For this review, take the finished solid that the model builds, in its own axes (mm). A direction names the side the tool comes from. Coordinates: 2 decimals unless noted, no trailing zeros. Write each loop counter-clockwise with the first axis right and the second up, starting at its lowest first coordinate (ties: lowest second). Pieces come first, ordered by that corner, then holes. Notation, with made-up numbers: (-35, -22) - (-1, -22) arc R24 ccw to (-1, -8) - close; hole circle Ø11 at (-2.5, -2). An arc over 180 degrees is marked (long way). Write each question's results on one line, items separated by ' | '.
from build123d import *

# Parameters (mm, degrees)
F0_R           = 11.4851473357
F1_DEPTH       = 25.4
F2_R           = 14.0381408387
F3_DEPTH       = 38.354
F4_R           = 11.1184182472
F5_DEPTH       = 40.64
F6_R           = 11.1443418508
F7_DEPTH       = 25.4
F8_R           = 10.6779324927
F9_DEPTH       = 25.4
F10_W          = 48.1841601431
F10_H          = 38.3043847978
F11_DEPTH      = 13.97
F11_DEPTH_BACK = 13.97
F12_W          = 27.94
F12_H          = 23.4013380416
F13_DEPTH      = 63.5
F14_W          = 27.5632794946
F14_H          = 12.7333622493
F14_H_2        = 23.4013380416
F14_H_3        = 14.7006912157
F15_DEPTH      = 6.35
F16_W          = 7.2420062497
F16_H          = 45.677350834
F16_W_2        = 6.9660460576
F16_H_2        = 44.3694461137
F17_DEPTH      = 6.35
F18_W          = 55.1662780344
F18_H          = 23.233897984
F19_DEPTH      = 6.35
F20_W          = 48.7214699388
F20_H          = 6.8689957261
F20_W_2        = 48.6058108509
F20_H_2        = 7.6186433434
F21_DEPTH      = 6.35
F22_W          = 23.1224743262
F22_H          = 101.739127886
F23_DEPTH      = 23.622
F24_W          = 28.0196964741
F24_H          = 23.2863202691
F25_DEPTH      = 12.7
F26_W          = 22.5610751659
F26_H          = 2.6592202485
F26_H_2        = 23.2863202691
F27_DEPTH      = 12.7
F28_W          = 54.3520981446
F28_H          = 22.9060128331
F28_W_2        = 2.7293106541
F29_DEPTH      = 5.08
F30_W          = 4.3049231172
F30_H          = 22.9060128331
F30_W_2        = 4.9764737487
F31_DEPTH      = 10.16
F32_W          = 22.9060128331
F32_H          = 2.5616861427
F33_DEPTH      = 2.54
F34_W          = 22.9060128331
F34_H          = 2.7740425909
F35_DEPTH      = 2.54
F36_R          = 10.668
F37_DEPTH      = 40.64
F38_R          = 3.2231915419
F39_DEPTH      = 22.86
F40_R          = 2.0835322845
F41_DEPTH      = 2.54
F42_R          = 5.3868280623
F43_DEPTH      = 7.62


with BuildPart() as f1:
    # F0 (on Top) → F1 (new body)
    with BuildSketch(Plane.XY):
        Circle(F0_R)
    extrude(amount=F1_DEPTH)


with BuildPart() as f3:
    # F2 (on Top) → F3 (new body)
    with BuildSketch(Plane.XY):
        Circle(F2_R)
    extrude(amount=F3_DEPTH)


with BuildPart() as f5_tool:
    # F4 (on Top) → F5 (new body)
    with BuildSketch(Plane.XY):
        Circle(F4_R)
    extrude(amount=F5_DEPTH)


with BuildPart() as f1_1:
    add(f1.part)

    # F5: cut by f5_tool
    add(f5_tool.part, mode=Mode.SUBTRACT)



with BuildPart() as f3_1:
    add(f3.part)

    # F5: cut by f5_tool
    add(f5_tool.part, mode=Mode.SUBTRACT)


with BuildPart() as f7:
    # F6 (on Top) → F7 (new body)
    with BuildSketch(Plane.XY):
        Circle(F6_R)
    extrude(amount=-F7_DEPTH)

    # F8 (on face) → F9 (cut)
    with BuildSketch(Plane(origin=(0, 0, -25.4), x_dir=(1, 0, 0), z_dir=(0, 0, -1))):
        Circle(F8_R)
    extrude(amount=-F9_DEPTH, mode=Mode.SUBTRACT)


with BuildPart() as f1_2:
    add(f1_1.part)

    add(f3_1.part)  # F11 merges F3

    add(f7.part)  # F11 merges F7
    # F10 (on Right) → F11 (join, two sides)
    with BuildSketch(Plane.YZ) as f11_sk:
        with Locations((-24.0920800716, 19.1521923989)):
            Rectangle(F10_W, F10_H)
    extrude(amount=F11_DEPTH)
    extrude(f11_sk.sketch, amount=-F11_DEPTH_BACK)

    # F12 (on face) → F13 (join)
    with BuildSketch(Plane.XY.offset(38.3043847978)):
        with Locations((0, -36.4834911223)):
            Rectangle(F12_W, F12_H)
    extrude(amount=F13_DEPTH)

    # F14 (on face) → F15 (join)
    with BuildSketch(Plane.XY.offset(101.8043847978)):
        with Locations((0, -18.4161409769)):
            Rectangle(F14_W, F14_H)
        with Locations((0, -36.4834911223)):
            Rectangle(F14_W, F14_H_2)
        with Locations((0, -55.534505751)):
            Rectangle(F14_W, F14_H_3)
    extrude(amount=F15_DEPTH)

    # F16 (on face) → F17 (cut)
    with BuildSketch(Plane.XY.offset(108.1543847978)):
        with Locations((5.9133009054, -37.9796130583)):
            Rectangle(F16_W, F16_H)
        with Locations((-8.0874641426, -37.8289176151)):
            Rectangle(F16_W_2, F16_H_2)
    extrude(amount=-F17_DEPTH, mode=Mode.SUBTRACT)

    # F18 (on face) → F19 (join)
    with BuildSketch(Plane.XY.offset(108.1543847978)):
        with Locations((0, -36.3346077502)):
            Rectangle(F18_W, F18_H)
    extrude(amount=F19_DEPTH)

    # F20 (on face) → F21 (cut)
    with BuildSketch(Plane.XY.offset(114.5043847978)):
        with Locations((0, -30.4647795856)):
            Rectangle(F20_W, F20_H)
        with Locations((0, -41.8227724731)):
            Rectangle(F20_W_2, F20_H_2)
    extrude(amount=-F21_DEPTH, mode=Mode.SUBTRACT)

    # F22 (on face) → F23 (cut)
    with BuildSketch(Plane.XZ.offset(48.1841601431)):
        with Locations((0, 50.869563943)):
            Rectangle(F22_W, F22_H)
    extrude(amount=-F23_DEPTH, mode=Mode.SUBTRACT)

    # F24 (on face) → F25 (join)
    with BuildSketch(Plane.XY.offset(114.5043847978)):
        with Locations((0, -36.3608188927)):
            Rectangle(F24_W, F24_H)
    extrude(amount=F25_DEPTH)

    # F26 (on face) → F27 (cut)
    with BuildSketch(Plane.XY.offset(127.2043847978)):
        with Locations((0, -49.3335891515)):
            Rectangle(F26_W, F26_H)
        with Locations((0, -36.3608188927)):
            Rectangle(F26_W, F26_H_2)
    extrude(amount=-F27_DEPTH, mode=Mode.SUBTRACT)

    # F28 (on face) → F29 (join)
    with BuildSketch(Plane.XY.offset(127.2043847978)):
        with Locations((-15.8955114894, -36.5509726107)):
            Rectangle(F28_W, F28_H)
        with Locations((12.64519291, -36.5509726107)):
            Rectangle(F28_W_2, F28_H)
    extrude(amount=F29_DEPTH)

    # F30 (on face) → F31 (join)
    with BuildSketch(Plane.XY.offset(132.2843847978)):
        with Locations((-40.9190990031, -36.5509726107)):
            Rectangle(F30_W, F30_H)
        with Locations((11.5216113627, -36.5509726107)):
            Rectangle(F30_W_2, F30_H)
    extrude(amount=F31_DEPTH)

    # F32 (on face) → F33 (join)
    with BuildSketch(Plane(origin=(9.0333744884, 0, 0), x_dir=(0, -1, 0), z_dir=(-1, 0, 0))):
        with Locations((36.5509726107, 141.1635417265)):
            Rectangle(F32_W, F32_H)
    extrude(amount=F33_DEPTH)

    # F34 (on face) → F35 (join)
    with BuildSketch(Plane.YZ.offset(-38.7666374445)):
        with Locations((-36.5509726107, 141.0573635024)):
            Rectangle(F34_W, F34_H)
    extrude(amount=F35_DEPTH)

    # F36 (on Top) → F37 (cut)
    with BuildSketch(Plane.XY):
        Circle(F36_R)
    extrude(amount=F37_DEPTH, mode=Mode.SUBTRACT)

    # F38 (on Front) → F39 (join)
    with BuildSketch(Plane.XZ):
        with Locations((0, 18.5866560787)):
            Circle(F38_R)
    extrude(amount=-F39_DEPTH)

    # F40 (on face) → F41 (join)
    with BuildSketch(Plane(origin=(0, 22.86, 0), x_dir=(-1, 0, 0), z_dir=(0, 1, 0))):
        with Locations((0, 18.5866560787)):
            Circle(F40_R)
    extrude(amount=F41_DEPTH)

    # F42 (on face) → F43 (join)
    with BuildSketch(Plane(origin=(0, 25.4, 0), x_dir=(-1, 0, 0), z_dir=(0, 1, 0))):
        with Locations((0, 18.5866560787)):
            Circle(F42_R)
    extrude(amount=F43_DEPTH)


solid = f1_2.part
Q1. Wall thickness on line 1 along X through (y, z) = (-54.5, 108); line 2 along Y through (x, z) = (0, 23); line 3 along Y through (x, z) = (0, 30): over which ranges is each line inside the solid? List them lowest first. Write a range as from..to.
Results found:
line 1: -13.78..-11.57, -4.6..2.29, 9.53..13.78 | line 2: -24.56..-10.67, 11.12..14.04, 25.4..33.02 | line 3: -24.56..-10.67, 11.12..14.04
Q2. Mouldability with a two-part tool opening along Y and no side actions: class faces 1 (the face through (-1.447, 11.024, 14.647)), 2 (the face through (-22, -36, 108.154)), 3 (the face through (-10, -48.004, 130)) as pulls with the +Y half, pulls with the -Y half, needs draft (parallel to the pull), parting line crosses it, or undercut.
Results found:
face 1: undercut | face 2: needs draft | face 3: pulls with the -Y half
Q3. Take a section at B-B on x = 21. State the section outline as (y, z) points, plus the area to 3 significant figures.
Results found:
outline: (-47.95, 108.15) - (-45.63, 108.15) - (-45.63, 114.5) - (-47.95, 114.5) - close; (-38.01, 108.15) - (-33.9, 108.15) - (-33.9, 114.5) - (-38.01, 114.5) - close; (-27.03, 108.15) - (-24.72, 108.15) - (-24.72, 114.5) - (-27.03, 114.5) - close | area: 55.5 mm2
Q4. Take a section at A-A on z = 121.5. State the section outline as (x, y) points, plus the area to 3 significant figures.
Results found:
outline: (-14.01, -48) - (-11.28, -48) - (-11.28, -24.72) - (-14.01, -24.72) - close; (11.28, -48) - (14.01, -48) - (14.01, -24.72) - (11.28, -24.72) - close | area: 127 mm2
Q5. Take a section at D-D on x = 0. State how many separate pieces and enclosed holes the cut face has, plus the area to 3 significant figures.
Results found:
separate pieces: 4 | enclosed holes: 0 | area: 1,390 mm2
Q6. For pin 1 (11.5 mm diameter, centred on x = -3.5, y = -10, fed in from +Z); pin 2 (4.5 mm diameter, centred on x = 5, y = -37, fed in from -Z); pin 3 (6 mm diameter, centred on x = 16.5, z = 102.5, fed in from -Y); pin 4 (10 mm diameter, centred on x = 1, y = -21, fed in from +Z), all flat-tipped, find the tip position at first contact; note any pin that passes through.
Results found:
pin 1: z = 108.15 | pin 2: z = 101.74 | pin 3: y = -62.88 | pin 4: z = 132.28
Q7. For faces 4 (the face through (24.303, -42, 111)), 5 (the face through (9.033, -37, 136)), 6 (the face through (0, -38.013, 111)), list the 3-axis set-ups (+Z, -Z, +X, -X, +Y, -Y) from which the entire face can be reached by the end or side of a thin tool; tool diameter is ignored.
Results found:
face 4: +Z, -Z | face 5: +Y, -Y | face 6: none
